Geometry check sheet. Reference: the model listing, model coordinates, mm. A direction names the side the tool comes from. Round coordinates to 2 decimals unless told otherwise and drop trailing zeros. Order: outer loops, then holes, each group sorted by start corner. A loop starts at its lowest first (then second) coordinate and runs counter-clockwise, first axis right, second up. Notation, with made-up numbers: (45, 20.5) -> (55, 20.5) arc R12 cw to (55, 40.5) -> close; hole circle Ø1 at (-19.75, 74). An arc over 180 degrees is marked (long way). Use a Markdown table: item, result. Add a question column.
Item 1: Sectioned sample at B-B, the plane x = 37. Record the cut outline in (y, z), and give its area (3 significant figures).
Item 2: Mould release check, pull along Z, two halves, no side actions. Record for faces 4 (the flat face through (4.3, 3, -49)), 5 (the flat face through (53.7, 3, -49)), 6 (the flat face through (28, 3, -2.3)): pulls with the +Z half, pulls with the -Z half, needs draft (parallel to the pull), parting line crosses it, or undercut.
Item 3: Sectioned sample at A-A, the plane z = -76. Record the cut outline in (x, y), and give its area (3 significant figures).
Item 4: Sectioned sample at C-C, the plane y = 3.6. Record the cut outline in (x, z).
Item 5: Set-up check for faces 1 (the flat face through (28, 3, -94.7)), 2 (the flat face through (28, 3, -96.7)), 3 (the flat face through (2.3, 3, -50)): record each of +Z, -Z, +X, -X, +Y, -Y from which the full face is reachable in a straight line by a thin tool's end or side.
Item 6: Gauge pin test, flat ends, axial feed: pin 1 Ø14 at (x, z) = (21, -28.5) entering from +Y; pin 2 Ø1.5 at (x, y) = (29, 3) entering from -Z; pin 3 Ø1.5 at (x, y) = (24, 4) entering from +Z. Record the tip position at first contact, or that the pin passes through.
Item 7: Material ranges on probe 1 along X at (y, z) = (3.15, -15.5); probe 2 along Z at (x, y) = (45, 3.7); probe 3 along Y at (x, z) = (43, -16.5), recorded low to high. Write a range as [from, to].
Autodesk Fusion 360 part; units mm, degrees
sketch "Boceto1" plane through (0, 0, 0) normal (0, 1, 0) x (1, 0, 0)
  line L0 (0, 0) -> (56, 0)
  line L1 (56, 0) -> (56, 99)
  line L2 (56, 99) -> (0, 99)
  line L3 (0, 99) -> (0, 0)
  dimension "d1" = 99
  dimension "d2" = 56
extrude "Extruir1" add sketch "Boceto1" along normal blind 2
sketch "Boceto2" plane through (0, 2, 0) normal (0, 1, 0) x (-1, 0, 0)
  line L0 (0, -99) -> (0, 0)
  line L1 (0, 0) -> (-56, 0)
  line L2 (-56, 0) -> (-56, -99)
  line L3 (-56, -99) -> (0, -99)
  line L4 (-2.3, -96.7) -> (-2.3, -2.3)
  line L5 (-2.3, -2.3) -> (-53.7, -2.3)
  line L6 (-53.7, -2.3) -> (-53.7, -96.7)
  line L7 (-53.7, -96.7) -> (-2.3, -96.7)
  line L8 (-4.3, -94.7) -> (-51.7, -94.7)
  line L9 (-51.7, -94.7) -> (-51.7, -4.3)
  line L10 (-51.7, -4.3) -> (-4.3, -4.3)
  line L11 (-4.3, -4.3) -> (-4.3, -94.7)
  dimension "d5" = -2.3
  dimension "d6" = 2
  dimension "d7" = 2
  dimension "d8" = 2
  dimension "d9" = 2
extrude "Extruir2" add sketch "Boceto2" along normal blind 3 contours L4 L5 L6 L7
fillet "Empalme1" radius 1 4 edges at (2.3, 3.5, -96.7) (53.7, 3.5, -96.7) (53.7, 3.5, -2.3) (2.3, 3.5, -2.3)
Found:
| question | item | result |
|---|---|---|
| 1 | outline | (0, -99) -> (2, -99) -> (2, -96.7) -> (5, -96.7) -> (5, -94.7) -> (2, -94.7) -> (2, -4.3) -> (5, -4.3) -> (5, -2.3) -> (2, -2.3) -> (2, 0) -> (0, 0) -> close |
| 1 | area | 210 mm2 |
| 2 | face 4 | undercut |
| 2 | face 5 | needs draft |
| 2 | face 6 | pulls with the +Z half |
| 3 | outline | (0, 0) -> (56, 0) -> (56, 2) -> (53.7, 2) -> (53.7, 5) -> (51.7, 5) -> (51.7, 2) -> (4.3, 2) -> (4.3, 5) -> (2.3, 5) -> (2.3, 2) -> (0, 2) -> close |
| 3 | area | 124 mm2 |
| 4 | outline | (2.3, -95.7) arc R1 ccw to (3.3, -96.7) -> (52.7, -96.7) arc R1 ccw to (53.7, -95.7) -> (53.7, -3.3) arc R1 ccw to (52.7, -2.3) -> (3.3, -2.3) arc R1 ccw to (2.3, -3.3) -> close; hole (4.3, -94.7) -> (51.7, -94.7) -> (51.7, -4.3) -> (4.3, -4.3) -> close |
| 5 | face 1 | +Y |
| 5 | face 2 | -Z, +X, -X, +Y |
| 5 | face 3 | +Z, -Z, -X, +Y |
| 6 | pin 1 | stops at y = 2 |
| 6 | pin 2 | stops at z = -96.7 |
| 6 | pin 3 | stops at z = -2.3 |
| 7 | probe 1 | x = [2.3, 4.3], [51.7, 53.7] |
| 7 | probe 2 | z = [-96.7, -94.7], [-4.3, -2.3] |
| 7 | probe 3 | y = [0, 2] |
